Autodesk Inventor part; units mm, degrees
ref_plane "YZ Plane" through (0, 0, 0) normal (1, 0, 0) x (0, 1, 0)
ref_plane "XZ Plane" through (0, 0, 0) normal (0, 1, 0) x (-1, 0, 0)
ref_plane "XY Plane" through (0, 0, 0) normal (0, 0, 1) x (1, 0, 0)
sketch "Sketch1" plane through (0, 0, 0) normal (0, 0, 1) x (1, 0, 0)
  line L0 (-19.1729, 62.3255) -> (30.8271, 62.3255)
  line L1 (30.8271, 62.3255) -> (30.8271, -12.6745)
  line L2 (30.8271, -12.6745) -> (-19.1729, -12.6745)
  line L3 (-19.1729, -12.6745) -> (-19.1729, 62.3255)
  dimension "d0" = 50
  dimension "d1" = 75
extrude "Extrusion1" add sketch "Sketch1" along normal blind 25
sketch "Sketch2" plane through (0, 0, 25) normal (0, 0, 1) x (1, 0, 0)
  circle A0 centre (0.8271, 25.3255) radius 12.5
  point P0 (-19.1729, -12.6745)
  dimension "d4" = 20
  dimension "d5" = 25
  dimension "d8" = 38
extrude "Extrusion2" cut sketch "Sketch2" against normal up to surface (25 mm away)
properties part number "box"
Source: CAD feature listing. Evaluate the final solid. Frame: model axes, mm. Coordinates: 2 decimals unless noted, no trailing zeros. Loops run counter-clockwise (first coordinate to the right, second up) from the corner with the lowest first, then second, coordinate; pieces in that order, holes last. Notation, with made-up numbers: M -36.5,8.5 L -18.5,8.5 A28 cw -18.5,34.5 Z; hole C -38.75,25 d10. An arc over 180 degrees is marked long. Use a Markdown table: item, result. Add a question column.
Q1. Section query C-C, the plane z = 13. Return loops of the section in (x, y), and give its area (3 significant figures).
Q2. First-contact query: pin 1 (2 mm diameter, centred on x = 24.5, y = 19.5, fed in from -Z). Flat tip, straight axial feed; report the tip coordinate or a pass-through.
Q3. Material intervals for L1, parallel to X at y = 29, z = 16.75; L2, parallel to Y at x = 4, z = 19.5; L3, parallel to Y at x = 5, z = 16.25, sorted ascending.
Q4. Draft query along X for faces 1 (the cylindrical face through (-1.883, 13.123, 12.675)), 2 (the flat face through (6, -12.674, 12)), 3 (the flat face through (30.827, 25, 12)), 4 (the flat face through (-19.173, 24, 12)). Return one class per face: pulls with the +X half, pulls with the -X half, needs draft (parallel to the pull), parting line crosses it, or undercut.
Q5. Section query A-A, the plane y = 33. Return loops of the section in (x, z), and give its area (3 significant figures).
Q6. Section query B-B, the plane x = -1. Return loops of the section in (y, z).
Result:
| question | item | result |
|---|---|---|
| 1 | outline | M -19.17,-12.67 L 30.83,-12.67 L 30.83,62.33 L -19.17,62.33 Z; hole C 0.83,25.33 d25 |
| 1 | area | 3,260 mm2 |
| 2 | pin 1 | stops at z = 0 |
| 3 | L1 | x = -19.17 to -11.12, 12.77 to 30.83 |
| 3 | L2 | y = -12.67 to 13.23, 37.42 to 62.33 |
| 3 | L3 | y = -12.67 to 13.54, 37.11 to 62.33 |
| 4 | face 1 | undercut |
| 4 | face 2 | needs draft |
| 4 | face 3 | pulls with the +X half |
| 4 | face 4 | pulls with the -X half |
| 5 | outline | M -19.17,0 L -9.04,0 L -9.04,25 L -19.17,25 Z; M 10.69,0 L 30.83,0 L 30.83,25 L 10.69,25 Z |
| 5 | area | 757 mm2 |
| 6 | outline | M -12.67,0 L 12.96,0 L 12.96,25 L -12.67,25 Z; M 37.69,0 L 62.33,0 L 62.33,25 L 37.69,25 Z |
